Could you check a few things on this model? Use its own coordinates, in mm. Face numbers are marked on the shaded views. A direction names the side the tool comes from. Coordinates: 2 decimals unless noted, no trailing zeros. Order: outer loops, then holes, each group sorted by start corner. A loop starts at its lowest first (then second) coordinate and runs counter-clockwise, first axis right, second up. Notation, with made-up numbers: (23, 27.5) -> (51, 27.5) arc R27 cw to (51, 55.5) -> close; hole circle Ø11 at (77.25, -27.75). An arc over 180 degrees is marked (long way). Use a Markdown table: item, result. Add a question column.
1) If we section it at A-A (x = 0): Write out the boundary of the cut face in (y, z).
2) Which directions (+Z, -Z, +X, -X, +Y, -Y) give clear straight access to the entire face, cutting with the end or side of a thin tool? Please do the marked faces 4, 5, 6, 7 and 8.
3) Thinking about a two-plate mould opening in Y: for the marked faces 1, 2 and 3, which applies, +Y half, -Y half, draft (parallel to the pull), parting line (faces both ways), or undercut?
4) If I drill on L1, parallel to Z at x = 0, y = 24; L2, parallel to Z at x = 0, y = -2.75; L3, parallel to X at y = 1, z = 3, over which ranges is the centre line in solid material (lowest first)? Write a range as [from, to].
5) Will these pins go through, and if not, where does the flat tip stop? pin 1 Ø1 at (x, z) = (7, -4.5) entering from -Y; pin 2 Ø9.5 at (y, z) = (86.5, 2.5) entering from -X; pin 3 Ø10.5 at (y, z) = (90.55, 0) entering from +X.
6) If we section it at C-C (z = -1.25): Give the number of separate pieces and of enclosed holes in the cut face, plus the area to 3 significant figures.
7) If we section it at B-B (y = -3.5): Write out the boundary of the cut face in (x, z).
8) If we section it at D-D (y = 40.5): Write out the boundary of the cut face in (x, z).
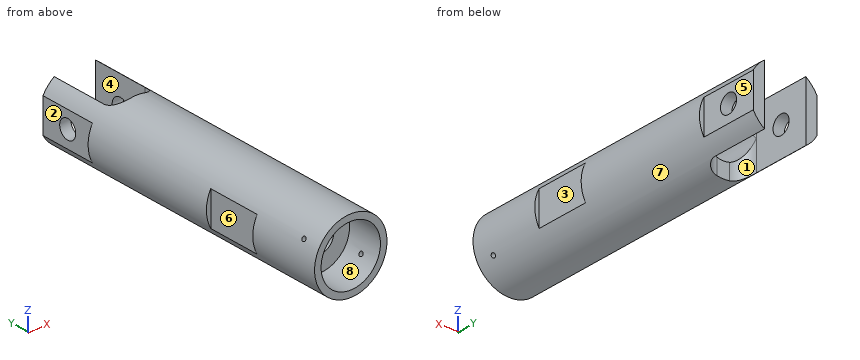
```python
from build123d import *

# Parameters (mm, degrees)
SKETCH1_R                                     = 12.7
SKETCH1_R_2                                   = 4.826
SOCKET_HEAD_STOP_DEPTH                        = 5.08
SKETCH2_R                                     = 12.7
SKETCH2_R_2                                   = 7.239
MAIN_BODY_DEPTH                               = 100.70719
SKETCH6_R                                     = 3.302
ROD_END_MOUNTING_HOLES_DEPTH                  = 13.7
ROD_END_MOUNTING_HOLES_DEPTH_BACK             = 13.7
SKETCH3_W                                     = 1.524
SKETCH3_H                                     = 19.05
SKETCH3_H_2                                   = 20.32
ROD_END_BODY_HOLES_AND_WRENCH_CUTS_DEPTH      = 13.7000001
ROD_END_BODY_HOLES_AND_WRENCH_CUTS_DEPTH_BACK = 13.7000001
SKETCH4_R                                     = 12.7
SKETCH4_R_2                                   = 10.414
RACK_COVER_DEPTH                              = 12.7
SKETCH7_R                                     = 0.762
SAFETY_WIRE_HOLES_DEPTH                       = 18.348522765
SAFETY_WIRE_HOLES_DEPTH_BACK                  = 18.348522765


with BuildPart() as part:
    # Sketch1 → Socket Head Stop (new body)
    with BuildSketch(Plane(origin=(0, 0, 0), x_dir=(1, 0, 0), z_dir=(0, 1, 0))):
        Circle(SKETCH1_R)
        Circle(SKETCH1_R_2, mode=Mode.SUBTRACT)
    extrude(amount=SOCKET_HEAD_STOP_DEPTH)

    # Sketch2 → Main Body (add)
    with BuildSketch(Plane(origin=(0, 0, 0), x_dir=(1, 0, 0), z_dir=(0, 1, 0))):
        Circle(SKETCH2_R)
        Circle(SKETCH2_R_2, mode=Mode.SUBTRACT)
    extrude(amount=MAIN_BODY_DEPTH)

    # Sketch6 → Rod End Mounting Holes (cut, two sides)
    with BuildSketch(Plane(origin=(0, 0, 0), x_dir=(0, 0, -1), z_dir=(1, 0, 0))) as rod_end_mounting_holes_sk:
        with Locations((0, 90.54719)):
            Circle(SKETCH6_R)
    extrude(amount=ROD_END_MOUNTING_HOLES_DEPTH, mode=Mode.SUBTRACT)
    extrude(rod_end_mounting_holes_sk.sketch, amount=-ROD_END_MOUNTING_HOLES_DEPTH_BACK, mode=Mode.SUBTRACT)

    # Sketch3 → Rod End Body Holes And Wrench Cuts (cut, two sides)
    with BuildSketch(Plane.XY) as rod_end_body_holes_and_wrench_cuts_sk:
        with BuildLine():
            Line((7.239, 100.70719), (-7.239, 100.70719))
            Line((-7.239, 100.70719), (-7.239, 80.38719))
            ThreePointArc((-7.239, 80.38719), (-5.751102448, 76.795087552), (-2.159, 75.30719))
            Line((-2.159, 75.30719), (2.159, 75.30719))
            ThreePointArc((2.159, 75.30719), (5.751102448, 76.795087552), (7.239, 80.38719))
            Line((7.239, 80.38719), (7.239, 100.70719))
        make_face()
        with Locations((11.938, 22.225)):
            Rectangle(SKETCH3_W, SKETCH3_H)
        with Locations((-11.938, 90.54719)):
            Rectangle(SKETCH3_W, SKETCH3_H_2)
        with Locations((11.938, 90.54719)):
            Rectangle(SKETCH3_W, SKETCH3_H_2)
        with Locations((-11.938, 22.225)):
            Rectangle(SKETCH3_W, SKETCH3_H)
    extrude(amount=ROD_END_BODY_HOLES_AND_WRENCH_CUTS_DEPTH, mode=Mode.SUBTRACT)
    extrude(rod_end_body_holes_and_wrench_cuts_sk.sketch, amount=-ROD_END_BODY_HOLES_AND_WRENCH_CUTS_DEPTH_BACK, mode=Mode.SUBTRACT)

    # Sketch4 → Rack Cover (add)
    with BuildSketch(Plane.XZ):
        Circle(SKETCH4_R)
        Circle(SKETCH4_R_2, mode=Mode.SUBTRACT)
    extrude(amount=RACK_COVER_DEPTH)

    # Sketch7 → Safety Wire Holes (cut, two sides)
    with BuildSketch(Plane(origin=(0, 0, 0), x_dir=(0, 1, 0), z_dir=(-0.866025404, 0, 0.5))) as safety_wire_holes_sk:
        with Locations((-6.35, 0)):
            Circle(SKETCH7_R)
    extrude(amount=SAFETY_WIRE_HOLES_DEPTH, mode=Mode.SUBTRACT)
    extrude(safety_wire_holes_sk.sketch, amount=-SAFETY_WIRE_HOLES_DEPTH_BACK, mode=Mode.SUBTRACT)


solid = part.part
```
Answer sheet:
| question | item | result |
|---|---|---|
| 1 | outline | (-12.7, -12.7) -> (75.31, -12.7) -> (75.31, -7.24) -> (5.08, -7.24) -> (5.08, -4.83) -> (0, -4.83) -> (0, -10.41) -> (-12.7, -10.41) -> close; (-12.7, 10.41) -> (0, 10.41) -> (0, 4.83) -> (5.08, 4.83) -> (5.08, 7.24) -> (75.31, 7.24) -> (75.31, 12.7) -> (-12.7, 12.7) -> close |
| 2 | face 4 | +Z, -Z, +Y |
| 2 | face 5 | +Z, -Z, +X, +Y |
| 2 | face 6 | +Z, -Z, -X |
| 2 | face 7 | +Y, -Y |
| 2 | face 8 | -Y |
| 3 | face 1 | +Y half |
| 3 | face 2 | draft |
| 3 | face 3 | undercut |
| 4 | L1 | [-12.7, -7.24], [7.24, 12.7] |
| 4 | L2 | [-12.7, -10.41], [10.41, 12.7] |
| 4 | L3 | [-12.34, -3.78], [3.78, 12.34] |
| 5 | pin 1 | y = 0 |
| 5 | pin 2 | x = -11.18 |
| 5 | pin 3 | x = 11.18 |
| 6 | separate pieces | 4 |
| 6 | enclosed holes | 0 |
| 6 | area | 1,030 mm2 |
| 7 | outline | circle Ø25.4 at (0, 0); hole circle Ø20.83 at (0, 0) |
| 8 | outline | circle Ø25.4 at (0, 0); hole circle Ø14.48 at (0, 0) |
